```python
from build123d import *

# Parameters (mm, degrees)
SKETCH1_W                = 55.88
SKETCH1_H                = 55.88
BOSS_EXTRUDE1_DEPTH      = 50.8
SKETCH2_W                = 43.18
SKETCH2_H                = 38.1
CUT_EXTRUDE1_DEPTH       = 56.88
SKETCH3_W                = 43.18
SKETCH3_H                = 38.1
CUT_EXTRUDE2_DEPTH       = 56.88
SKETCH4_R                = 1.75
SKETCH4_W                = 25.4
SKETCH4_H                = 25.4
CUT_EXTRUDE3_DEPTH       = 44.45
BOSS_EXTRUDE2_DEPTH      = 3.175
BOSS_EXTRUDE2_DEPTH_BACK = 3.175
SKETCH10_W               = 9.525
SKETCH10_H               = 3.175
BOSS_EXTRUDE5_DEPTH      = 55.88
SKETCH11_R               = 1.75
CUT_EXTRUDE4_DEPTH       = 48.625


with BuildPart() as part:
    # Sketch1 → Boss-Extrude1 (new body)
    with BuildSketch(Plane(origin=(0, 0, 0), x_dir=(1, 0, 0), z_dir=(0, 1, 0))):
        with Locations((27.94, 27.94)):
            Rectangle(SKETCH1_W, SKETCH1_H)
    extrude(amount=BOSS_EXTRUDE1_DEPTH)

    # Sketch2 → Cut-Extrude1 (cut, through all)
    with BuildSketch(Plane.XY):
        with Locations((27.94, 25.4)):
            Rectangle(SKETCH2_W, SKETCH2_H)
    extrude(amount=-CUT_EXTRUDE1_DEPTH, mode=Mode.SUBTRACT)

    # Sketch3 → Cut-Extrude2 (cut, through all)
    with BuildSketch(Plane(origin=(55.88, 0, 0), x_dir=(0, 0, -1), z_dir=(1, 0, 0))):
        with Locations((27.94, 25.4)):
            Rectangle(SKETCH3_W, SKETCH3_H)
    extrude(amount=-CUT_EXTRUDE2_DEPTH, mode=Mode.SUBTRACT)

    # Sketch4 → Cut-Extrude3 (cut)
    with BuildSketch(Plane(origin=(0, 50.8, 0), x_dir=(1, 0, 0), z_dir=(0, 1, 0))):
        with Locations((43.44, 43.44)):
            Circle(SKETCH4_R)
        with Locations((43.44, 12.44)):
            Circle(SKETCH4_R)
        with Locations((12.44, 12.44)):
            Circle(SKETCH4_R)
        with Locations((12.44, 43.44)):
            Circle(SKETCH4_R)
        with Locations((27.94, 27.94)):
            Rectangle(SKETCH4_W, SKETCH4_H)
    extrude(amount=-CUT_EXTRUDE3_DEPTH, mode=Mode.SUBTRACT)

    # Sketch5 → Cut-Revolve1 (revolve, cut)
    with BuildSketch(Plane(origin=(12.44, 0, 0), x_dir=(0, 0, -1), z_dir=(1, 0, 0))):
        Polygon((43.44, 50.8), (40.138, 50.8), (43.44, 47.498), align=None)
    revolve(axis=Axis((12.44, 47.498, -43.44), (0, 1, 0)), mode=Mode.SUBTRACT)

    # Sketch6 → Cut-Revolve2 (revolve, cut)
    with BuildSketch(Plane(origin=(12.44, 0, 0), x_dir=(0, 0, -1), z_dir=(1, 0, 0))):
        Polygon((12.44, 50.8), (9.138, 50.8), (12.44, 47.498), align=None)
    revolve(axis=Axis((12.44, 47.498, -12.44), (0, 1, 0)), mode=Mode.SUBTRACT)

    # Sketch7 → Cut-Revolve3 (revolve, cut)
    with BuildSketch(Plane(origin=(43.44, 0, 0), x_dir=(0, 0, -1), z_dir=(1, 0, 0))):
        Polygon((43.44, 50.8), (40.138, 50.8), (43.44, 47.498), align=None)
    revolve(axis=Axis((43.44, 47.498, -43.44), (0, 1, 0)), mode=Mode.SUBTRACT)

    # Sketch8 → Cut-Revolve4 (revolve, cut)
    with BuildSketch(Plane(origin=(43.44, 0, 0), x_dir=(0, 0, -1), z_dir=(1, 0, 0))):
        Polygon((12.44, 50.8), (9.138, 50.8), (12.44, 47.498), align=None)
    revolve(axis=Axis((43.44, 47.498, -12.44), (0, 1, 0)), mode=Mode.SUBTRACT)

    # Sketch9 → Boss-Extrude2 (add, two sides)
    with BuildSketch(Plane.XZ.offset(-44.45)) as boss_extrude2_sk:
        with BuildLine():
            Line((0, -40.64), (0, -15.24))
            ThreePointArc((0, -15.24), (-1.005581006, -19.499709497), (-3.81, -22.86))
            ThreePointArc((-3.81, -22.86), (-6.35, -27.94), (-3.81, -33.02))
            ThreePointArc((-3.81, -33.02), (-1.005581006, -36.380290503), (0, -40.64))
        make_face()
        with BuildLine():
            Line((55.88, -40.64), (55.88, -15.24))
            ThreePointArc((55.88, -15.24), (56.885581006, -19.499709497), (59.69, -22.86))
            ThreePointArc((59.69, -22.86), (62.23, -27.94), (59.69, -33.02))
            ThreePointArc((59.69, -33.02), (56.885581006, -36.380290503), (55.88, -40.64))
        make_face()
    extrude(amount=BOSS_EXTRUDE2_DEPTH)
    extrude(boss_extrude2_sk.sketch, amount=-BOSS_EXTRUDE2_DEPTH_BACK)

    # Sketch10 → Boss-Extrude5 (add)
    with BuildSketch(Plane.XY):
        with Locations((54.2925, 42.8625)):
            Rectangle(SKETCH10_W, SKETCH10_H)
        with Locations((1.5875, 42.8625)):
            Rectangle(SKETCH10_W, SKETCH10_H)
    extrude(amount=-BOSS_EXTRUDE5_DEPTH)

    # Sketch11 → Cut-Extrude4 (cut, through all)
    with BuildSketch(Plane(origin=(0, 47.625, 0), x_dir=(1, 0, 0), z_dir=(0, 1, 0))):
        with Locations((-3.81, 27.94)):
            Circle(SKETCH11_R)
        with Locations((59.69, 27.94)):
            Circle(SKETCH11_R)
    extrude(amount=-CUT_EXTRUDE4_DEPTH, mode=Mode.SUBTRACT)


solid = part.part
```
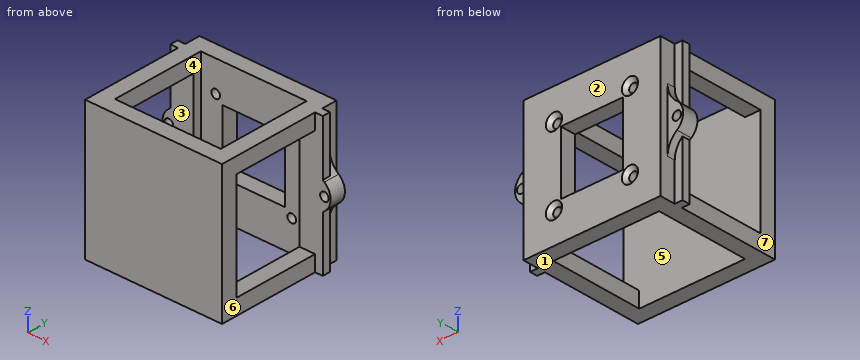
Design review of the part built by this model. Coordinates are the model's own, in mm. Face numbers are marked on the shaded views. A direction names the side the tool comes from. Round coordinates to 2 decimals unless told otherwise and drop trailing zeros. Write each loop counter-clockwise with the first axis right and the second up, starting at its lowest first coordinate (ties: lowest second). Pieces come first, ordered by that corner, then holes. Notation, with made-up numbers: (71, -10) -> (128, -10) arc R16 cw to (128, 19) -> close; hole circle Ø5 at (12.5, 59). An arc over 180 degrees is marked (long way). Write item = value, one per line. Start each with the question number.
1) Take a section at A-A, the plane x = 43.44. State the section outline as (y, z) points.
2) Clearance check with flat-ended pins moving along their axes: pin 1 (12 mm diameter, centred on y = 13.5, z = -48.5, fed in from -X); pin 2 (5.5 mm diameter, centred on x = 59.69, z = -27.94, fed in from +Y) (3 decimals); pin 3 (2.5 mm diameter, centred on y = 42.5, z = -40, fed in from +X) (3 decimals). State where each tip first meets the part, or that it passes through.
3) Take a section at D-D, the plane z = -43.44. State the section outline as (x, y) points (3 decimals).
4) Tool access review of the marked faces 4, 5, 6 and 7: name each direction out of +Z, -Z, +X, -X, +Y, -Y from which nothing blocks a thin tool from reaching the whole face with its end or side.
5) Wall thickness on probe 1 along X at (y, z) = (47.1, -12.44); probe 2 along Z at (x, y) = (12.44, 45.4); probe 3 along Y at (x, z) = (47, -42): over which ranges is each line inside the solid? List them lowest first. Write a range as from..to.
6) Mouldability with a two-part tool opening along Z and no side actions: class the marked faces 1, 2 and 3 as +Z half, -Z half, draft (parallel to the pull), parting line (faces both ways), or undercut.
7) Take a section at B-B, the plane y = 8.5. State the section outline as (x, z) points.
8) Take a section at C-C, the plane y = 43.5. State the section outline as (x, z) points (3 decimals), plus the area to 3 significant figures.
Results list:
q1.outline = (0, -55.88) -> (6.35, -55.88) -> (6.35, 0) -> (0, 0) -> close; (44.45, -55.88) -> (50.8, -55.88) -> (50.8, -46.74) -> (49.25, -45.19) -> (44.45, -45.19) -> close; (44.45, -41.69) -> (49.25, -41.69) -> (50.8, -40.14) -> (50.8, -15.74) -> (49.25, -14.19) -> (44.45, -14.19) -> close; (44.45, -10.69) -> (49.25, -10.69) -> (50.8, -9.14) -> (50.8, 0) -> (44.45, 0) -> close
q2.pin_1 = 0
q2.pin_2 = 47.625
q2.pin_3 = 59.055
q3.outline = (-3.175, 41.275) -> (6.35, 41.275) -> (6.35, 44.45) -> (10.69, 44.45) -> (10.69, 49.248) -> (9.138, 50.8) -> (0, 50.8) -> (0, 44.45) -> (-3.175, 44.45) -> close; (0, 0) -> (55.88, 0) -> (55.88, 6.35) -> (0, 6.35) -> close; (14.19, 44.45) -> (41.69, 44.45) -> (41.69, 49.248) -> (40.138, 50.8) -> (15.742, 50.8) -> (14.19, 49.248) -> close; (45.19, 44.45) -> (49.53, 44.45) -> (49.53, 41.275) -> (59.055, 41.275) -> (59.055, 44.45) -> (55.88, 44.45) -> (55.88, 50.8) -> (46.742, 50.8) -> (45.19, 49.248) -> close
q4.face_4 = +Z, -Z
q4.face_5 = none
q4.face_6 = +Z, -Z, +X, -Y
q4.face_7 = +Z, -Z, -X, -Y
q5.probe_1 = 0..10.69, 14.19..41.69, 45.19..55.88
q5.probe_2 = -55.88..-45.19, -41.69..-14.19, -10.69..0
q5.probe_3 = 0..6.35, 44.45..50.8
q6.face_1 = -Z half
q6.face_2 = draft
q6.face_3 = undercut
q7.outline = (0, -55.88) -> (6.35, -55.88) -> (6.35, -49.53) -> (0, -49.53) -> close; (0, -6.35) -> (6.35, -6.35) -> (6.35, 0) -> (0, 0) -> close; (49.53, -55.88) -> (55.88, -55.88) -> (55.88, -49.53) -> (49.53, -49.53) -> close; (49.53, -6.35) -> (55.88, -6.35) -> (55.88, 0) -> (49.53, 0) -> close
q8.outline = (-3.81, -33.02) arc R9.525 cw to (-3.175, -33.54) -> (-3.175, -55.88) -> (6.35, -55.88) -> (6.35, 0) -> (-3.175, 0) -> (-3.175, -22.34) arc R9.525 cw to (-3.81, -22.86) arc R6.35 ccw to start; (49.53, -55.88) -> (59.055, -55.88) -> (59.055, -33.54) arc R9.525 cw to (59.69, -33.02) arc R6.35 ccw to (59.69, -22.86) arc R9.525 cw to (59.055, -22.34) -> (59.055, 0) -> (49.53, 0) -> close; hole circle Ø3.5 at (-3.81, -27.94); hole circle Ø3.5 at (59.69, -27.94)
q8.area = 1,090 mm²
